For this review, use the dimensioned drawing (mm, ordinates from the lowest corner) and the shaded views. A direction names the side the tool comes from. Coordinates: 2 decimals unless noted, no trailing zeros. Loops run counter-clockwise (first coordinate to the right, second up) from the corner with the lowest first, then second, coordinate; pieces in that order, holes last. Notation, with made-up numbers: (26, -11) - (31, -11) arc R18 ccw to (31, -7) - close; hole circle Ø10 at (57, 32). An arc over 180 degrees is marked (long way). Answer in a Markdown table with one row per item. Add a question column.
(1) We need section D-D on z = 0.4. Write out the cut boundary in (x, y).
(2) Machinability: for the marked faces 1, 2 and 3, which of the approach directions +Z, -Z, +X, -X, +Y, -Y give a long, thin tool a straight path to every point of the face, cutting with its end or side? Answer none if there is none.
(3) We need section C-C on x = 6.8. Write out the cut boundary in (y, z), plus the area to 3 significant figures.
(4) We need section B-B on z = 3.3. Write out the cut boundary in (x, y).
(5) For line 1 along Z through (x, y) = (10.16, 2.8); line 2 along Y through (x, z) = (8.5, 1.95); line 3 along Y through (x, z) = (12.25, 4.1), list the stretches that pass through material, from the lowest coordinate up.
(6) Mouldability with a two-part tool opening along Z and no side actions: class the marked faces 4, 5 and 6 as +Z half, -Z half, draft (parallel to the pull), parting line (faces both ways), or undercut.
(7) For P1, Ø1.5, axis at y = 15.5, z = 3, coming from the +X side; P2, Ø1.5, axis at x = 5.5, z = 2.5, coming from the -Y side; P3, Ø2, axis at y = 28, z = 1.5, coming from the +X side, all flat-tipped, find the tip position at first contact; note any pin that passes through.
(8) We need section A-A on x = 10.16. Write out the cut boundary in (y, z).
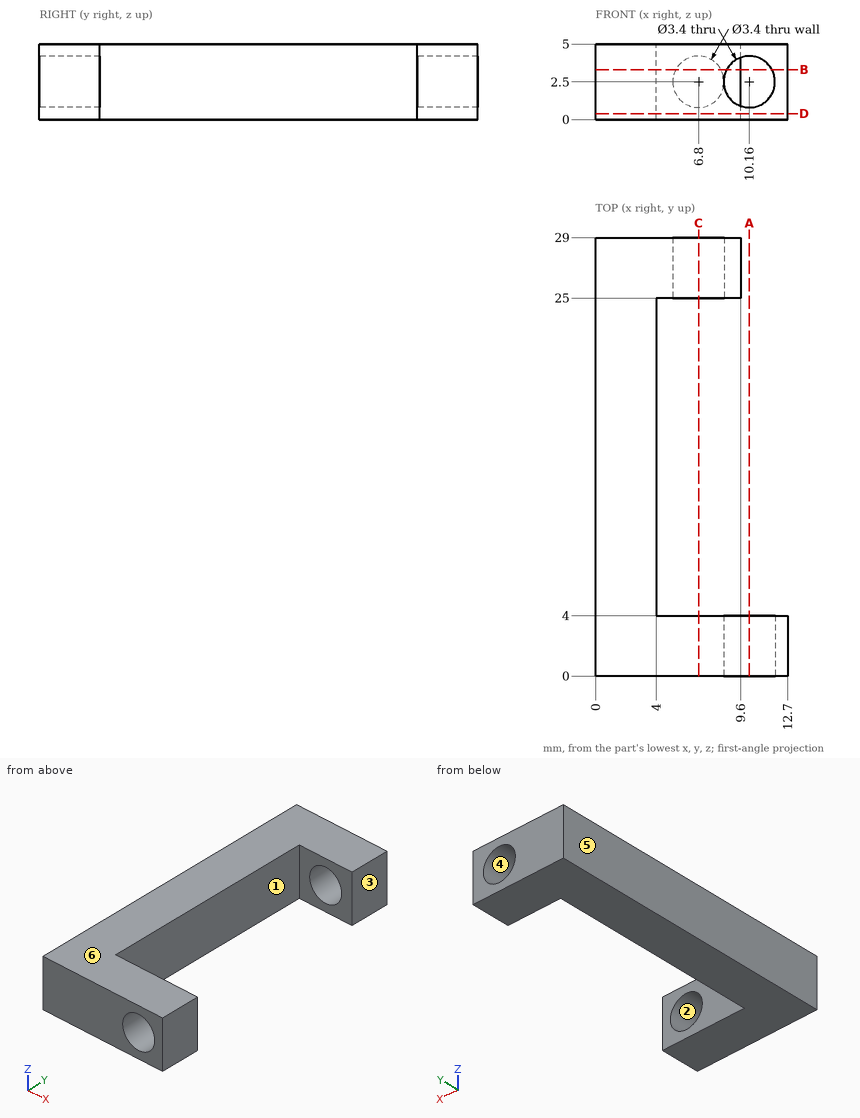
Outcome:
| question | item | result |
|---|---|---|
| 1 | outline | (0, 0) - (12.7, 0) - (12.7, 4) - (4, 4) - (4, 25) - (9.6, 25) - (9.6, 29) - (0, 29) - close |
| 2 | face 1 | +Z, -Z, +X |
| 2 | face 2 | -Y |
| 2 | face 3 | +Z, -Z, +X, +Y |
| 3 | outline | (0, 0) - (4, 0) - (4, 5) - (0, 5) - close; (25, 0) - (29, 0) - (29, 0.8) - (25, 0.8) - close; (25, 4.2) - (29, 4.2) - (29, 5) - (25, 5) - close |
| 3 | area | 26.4 mm² |
| 4 | outline | (0, 0) - (8.66, 0) - (8.66, 4) - (4, 4) - (4, 25) - (5.3, 25) - (5.3, 29) - (0, 29) - close; (8.3, 25) - (9.6, 25) - (9.6, 29) - (8.3, 29) - close; (11.66, 0) - (12.7, 0) - (12.7, 4) - (11.66, 4) - close |
| 5 | line 1 | 0 to 0.8, 4.2 to 5 |
| 5 | line 2 | 0 to 4, 25 to 29 |
| 5 | line 3 | 0 to 4 |
| 6 | face 4 | undercut |
| 6 | face 5 | draft |
| 6 | face 6 | +Z half |
| 7 | P1 | x = 4 |
| 7 | P2 | y = 0 |
| 7 | P3 | x = 9.6 |
| 8 | outline | (0, 0) - (4, 0) - (4, 0.8) - (0, 0.8) - close; (0, 4.2) - (4, 4.2) - (4, 5) - (0, 5) - close |
